Geometry check sheet. Reference: drawing and pictorial views, mm from the part's lowest x, y, z. A direction names the side the tool comes from. Give positions to 0.01 mm unless a question says otherwise; leave off trailing zeros. Order: outer loops, then holes, each group sorted by start corner. A loop starts at its lowest first (then second) coordinate and runs counter-clockwise, first axis right, second up. Notation, with made-up numbers: (74.25, -20) -> (78.25, -20) arc R15 ccw to (78.25, -5) -> close; hole circle Ø5 at (5, 10.5). An arc over 180 degrees is marked (long way). Write each question's results on one line, items separated by ' | '. Start each with the question number.
1. Cross-section at A-A, the plane x = 84.75. Enter the section's corners in (y, z), then the cut area to 3 significant figures.
2. Mould release check, pull along Z, two halves, no side actions. Record for the marked faces 1, 2, 3 and 4: +Z half, -Z half, draft (parallel to the pull), parting line (faces both ways), or undercut.
3. Cross-section at C-C, the plane z = 17.5. Enter the section's corners in (x, y).
4. Set-up check for the marked faces 5, 6, 7 and 8: record each of +Z, -Z, +X, -X, +Y, -Y from which the full face is reachable in a straight line by a thin tool's end or side.
5. Cross-section at B-B, the plane y = 11.75. Enter the section's corners in (x, z).
6. Cross-section at D-D, the plane y = 4.75. Enter the section's corners in (x, z), then the cut area to 3 significant figures.
7. Depth check by flat-ended pin: pin 1 Ø21 at (x, z) = (26, 17) entering from +Y; pin 2 Ø5.5 at (y, z) = (4.5, 3) entering from +X; pin 3 Ø5 at (y, z) = (8.5, 13) entering from +X; pin 4 Ø7.5 at (y, z) = (12, 17.5) entering from -X. Enter the tip coordinate at first touch or a pass-through.
8. Material ranges on L1, parallel to X at y = 0.45, z = 6.84; L2, parallel to Z at x = 84.75, y = 0.3; L3, parallel to Z at x = 63, y = 14.5, recorded low to high. Write a range as from..to.
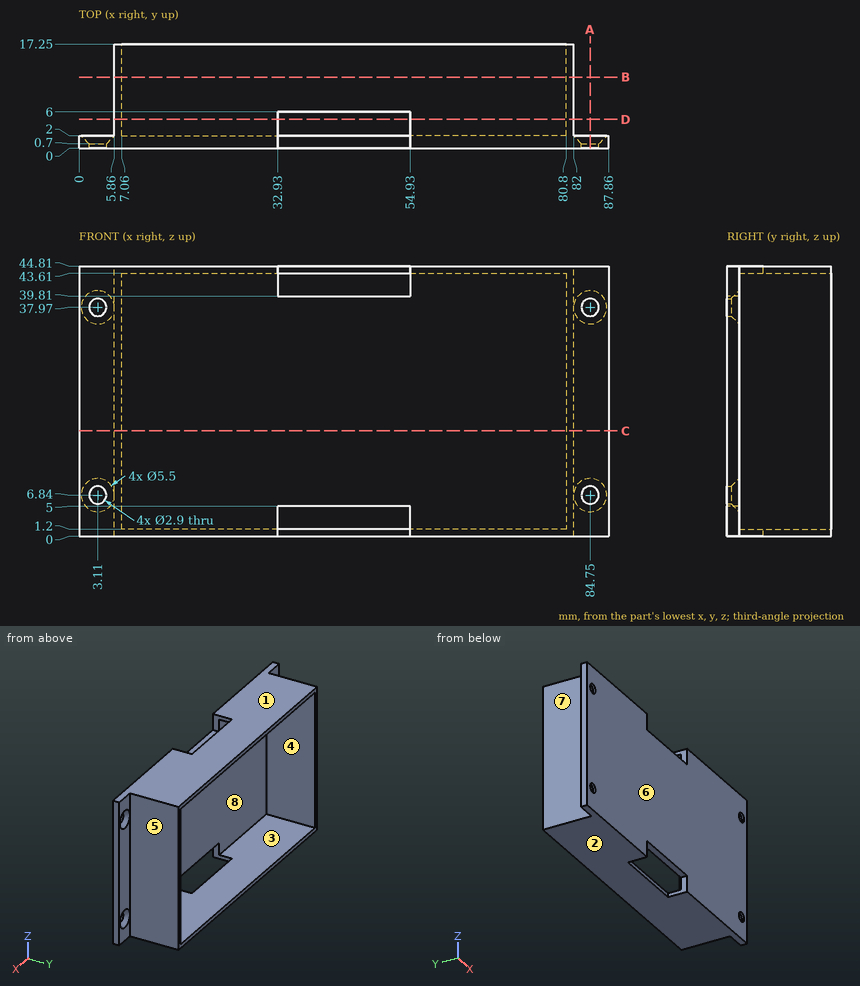
Results below:
1) outline: (0, 0) -> (2, 0) -> (2, 4.09) -> (0.7, 5.39) -> (0, 5.39) -> close; (0, 8.29) -> (0.7, 8.29) -> (2, 9.59) -> (2, 35.22) -> (0.7, 36.52) -> (0, 36.52) -> close; (0, 39.42) -> (0.7, 39.42) -> (2, 40.72) -> (2, 44.81) -> (0, 44.81) -> close | area: 74.6 mm²
2) face 1: +Z half | face 2: -Z half | face 3: undercut | face 4: undercut
3) outline: (0, 0) -> (87.86, 0) -> (87.86, 2) -> (82, 2) -> (82, 17.25) -> (80.8, 17.25) -> (80.8, 2) -> (7.06, 2) -> (7.06, 17.25) -> (5.86, 17.25) -> (5.86, 2) -> (0, 2) -> close
4) face 5: +Z, -Z, +X, +Y | face 6: +Z, -Z, +X, -X, -Y | face 7: +Z, -Z, -X, +Y | face 8: +Y
5) outline: (5.86, 0) -> (82, 0) -> (82, 44.81) -> (5.86, 44.81) -> close; hole (7.06, 1.2) -> (80.8, 1.2) -> (80.8, 43.61) -> (7.06, 43.61) -> close
6) outline: (5.86, 0) -> (32.93, 0) -> (32.93, 1.2) -> (7.06, 1.2) -> (7.06, 43.61) -> (32.93, 43.61) -> (32.93, 44.81) -> (5.86, 44.81) -> close; (54.93, 0) -> (82, 0) -> (82, 44.81) -> (54.93, 44.81) -> (54.93, 43.61) -> (80.8, 43.61) -> (80.8, 1.2) -> (54.93, 1.2) -> close | area: 232 mm²
7) pin 1: stops at y = 2 | pin 2: stops at x = 87.86 | pin 3: stops at x = 82 | pin 4: stops at x = 5.86
8) L1: x = 0..1.66, 4.56..83.3, 86.2..87.86 | L2: z = 0..5.39, 8.29..36.52, 39.42..44.81 | L3: z = 0..1.2, 43.61..44.81
